Verification items for this drawing (mm, ordinates from the low corner). A direction names the side the tool comes from. Give positions to 0.01 mm unless a question says otherwise; leave off trailing zeros. Order: outer loops, then holes, each group sorted by start corner. A loop starts at its lowest first (then second) coordinate and runs counter-clockwise, first axis right, second up. Notation, with made-up numbers: M 68,-32 L 111,-32 A25 ccw 111,4 Z; hole C 58,17.25 d2. An arc over 180 degrees is marked long. Answer as a JSON object with one key per item and string values.
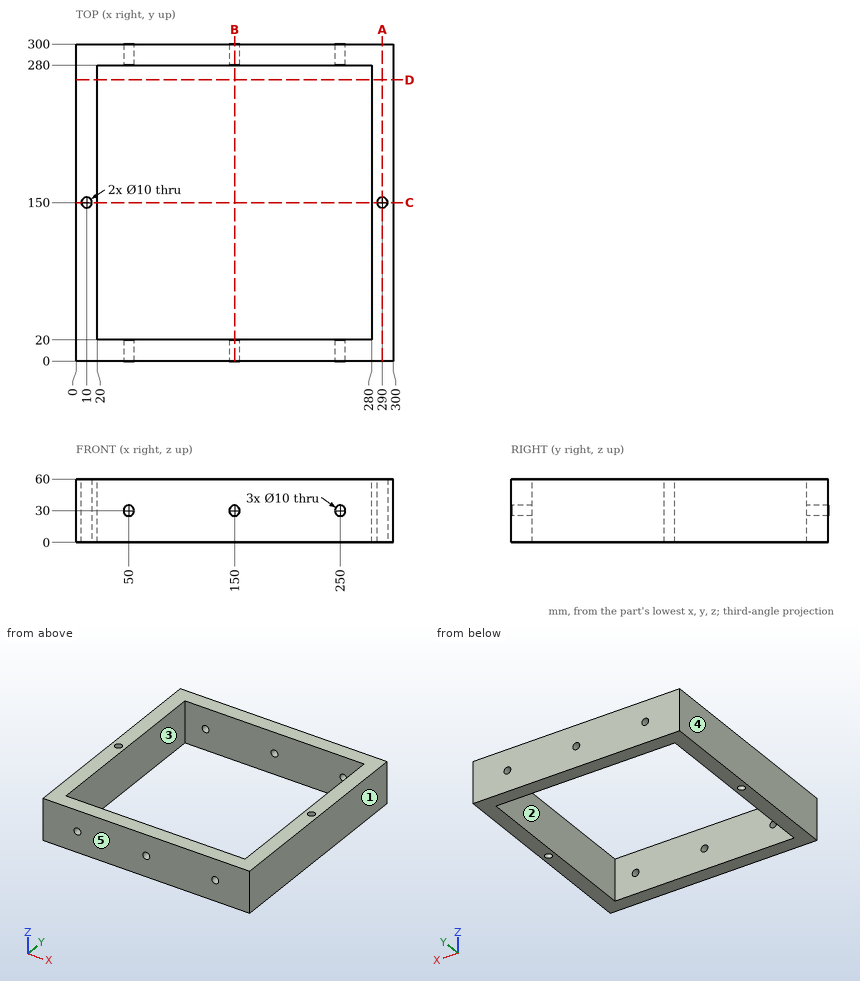
Q1. Section check C-C on y = 150. Record the cut outline in (x, z).
Resolved:
{"outline": "M 0,0 L 5,0 L 5,60 L 0,60 Z; M 15,0 L 20,0 L 20,60 L 15,60 Z; M 280,0 L 285,0 L 285,60 L 280,60 Z; M 295,0 L 300,0 L 300,60 L 295,60 Z"}
Q2. Release check for a two-part mould opening along Y. For the marked faces 3, 4 and 5 record: +Y half, -Y half, draft (parallel to the pull), parting line (faces both ways), or undercut.
Resolved:
{"face 3": "undercut", "face 4": "draft", "face 5": "-Y half"}
Q3. Tool access check on the marked faces 1 and 2. Record the directions out of +Z, -Z, +X, -X, +Y, -Y that give a thin tool (end or side, any length) a straight path to the whole face; none if there is none.
Resolved:
{"face 1": "+Z, -Z, +X, +Y, -Y", "face 2": "+Z, -Z"}
Q4. Section check A-A on x = 290. Record the cut outline in (y, z).
Resolved:
{"outline": "M 0,0 L 145,0 L 145,60 L 0,60 Z; M 155,0 L 300,0 L 300,60 L 155,60 Z"}
Q5. Material ranges on L1, parallel to Z at x = 250, y = 11.5; L2, parallel to Y at x = 60, z = 22, recorded low to high.
Resolved:
{"L1": "z = 0 to 25, 35 to 60", "L2": "y = 0 to 20, 280 to 300"}
Q6. Section check D-D on y = 266. Record the cut outline in (x, z), then the cut area to 3 significant figures.
Resolved:
{"outline": "M 0,0 L 20,0 L 20,60 L 0,60 Z; M 280,0 L 300,0 L 300,60 L 280,60 Z", "area": "2,400 mm²"}
Q7. Gauge pin test, flat ends, axial feed: pin 1 Ø4 at (x, z) = (265.5, 18.5) entering from -Y; pin 2 Ø6 at (x, y) = (10, 150) entering from -Z (1 decimal). Record the tip position at first contact, or that the pin passes through.
Resolved:
{"pin 1": "stops at y = 0", "pin 2": "passes through"}
Q8. Section check B-B on x = 150. Record the cut outline in (y, z).
Resolved:
{"outline": "M 0,0 L 20,0 L 20,25 L 0,25 Z; M 0,35 L 20,35 L 20,60 L 0,60 Z; M 280,0 L 300,0 L 300,25 L 280,25 Z; M 280,35 L 300,35 L 300,60 L 280,60 Z"}
